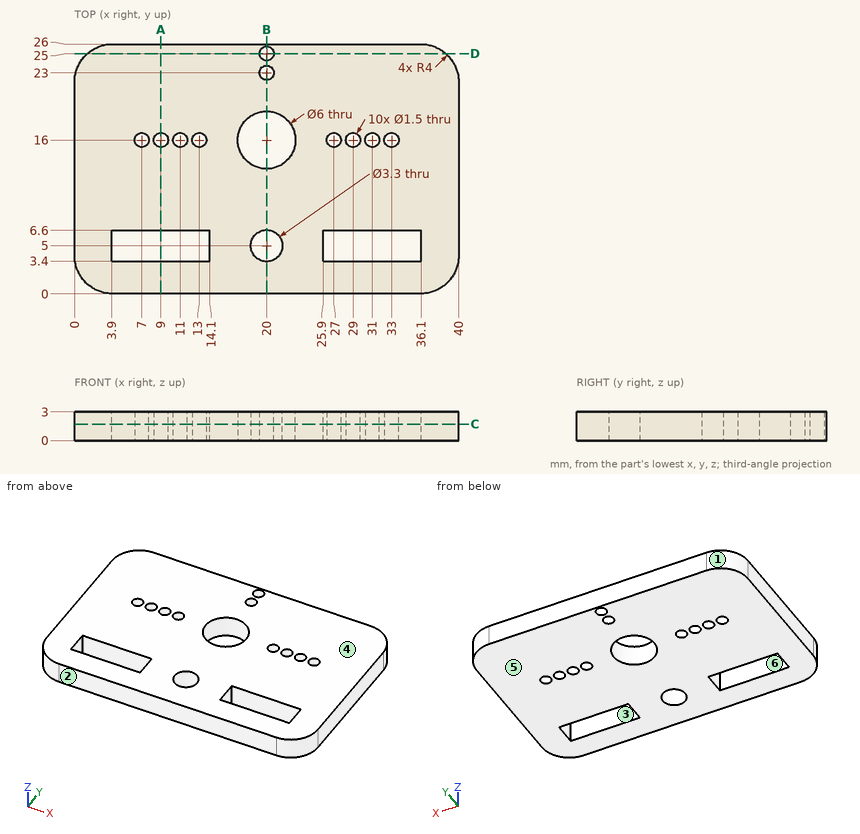
Print and shaded views of the part. All mm, measured from the part's lowest x, y and z. A direction names the side the tool comes from. Give positions to 0.01 mm unless a question says otherwise; leave off trailing zeros. Loops run counter-clockwise (first coordinate to the right, second up) from the corner with the lowest first, then second, coordinate; pieces in that order, holes last.
1) Saw through at B-B (x = 20). Write the cut outline in (y, z), plus the area to 3 significant figures.
2) Pull direction Y, two halves, no side cores. Call the marked faces 1, 2, 3 and 4: +Y half, -Y half, draft (parallel to the pull), parting line (faces both ways), or undercut.
3) Saw through at A-A (x = 9). Write the cut outline in (y, z).
4) Saw through at C-C (z = 1.7). Count the separate pieces of the cut face and the enclosed holes in it, plus the area to 3 significant figures.
5) Wall check: line 1 (Y direction, x = 13, z = 2.05); line 2 (Y direction, x = 20, z = 1.55); line 3 (Y direction, x = 4, z = 2.8). Give the ranges that are in metal, low to high.
6) Tool access for the marked faces 5 and 6: list every direction of +Z, -Z, +X, -X, +Y, -Y with a clear straight run to the whole face (end or side of a thin tool).
7) Flat gauge pin, fed straight in: pin 1 Ø1.7 at (x, y) = (33, 16) entering from -Z. Where does the tip first touch, or does it go through?
8) Saw through at D-D (y = 25). Write the cut outline in (x, z), plus the area to 3 significant figures.
Answer block:
1. outline: (0, 0) - (3.35, 0) - (3.35, 3) - (0, 3) - close; (6.65, 0) - (13, 0) - (13, 3) - (6.65, 3) - close; (19, 0) - (22.25, 0) - (22.25, 3) - (19, 3) - close; (23.75, 0) - (24.25, 0) - (24.25, 3) - (23.75, 3) - close; (25.75, 0) - (26, 0) - (26, 3) - (25.75, 3) - close
1. area: 41.1 mm2
2. face 1: +Y half
2. face 2: -Y half
2. face 3: undercut
2. face 4: draft
3. outline: (0, 0) - (3.4, 0) - (3.4, 3) - (0, 3) - close; (6.6, 0) - (15.25, 0) - (15.25, 3) - (6.6, 3) - close; (16.75, 0) - (26, 0) - (26, 3) - (16.75, 3) - close
4. separate pieces: 1
4. enclosed holes: 14
4. area: 906 mm2
5. line 1: y = 0 to 3.4, 6.6 to 15.25, 16.75 to 26
5. line 2: y = 0 to 3.35, 6.65 to 13, 19 to 22.25, 23.75 to 24.25, 25.75 to 26
5. line 3: y = 0 to 3.4, 6.6 to 26
6. face 5: -Z, +X, -X, +Y, -Y
6. face 6: +Z, -Z
7. pin 1: stops at z = 0
8. outline: (1.35, 0) - (19.25, 0) - (19.25, 3) - (1.35, 3) - close; (20.75, 0) - (38.65, 0) - (38.65, 3) - (20.75, 3) - close
8. area: 107 mm2
